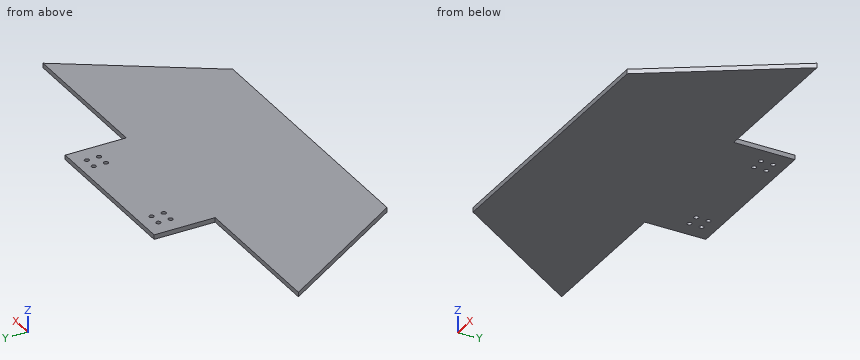
```python
from build123d import *

# Parameters (mm, degrees)
EXTRUDE_1_DEPTH     = 3
CUT_EXTRUDE_1_DEPTH = 10
SKETCH_3_R          = 1.5
CUT_EXTRUDE_2_DEPTH = 10


with BuildPart() as part:
    # 草图1 → 凸台-拉伸1 (new body)
    with BuildSketch(Plane.XY):
        Polygon((100, 0), (250, 0), (250, -30), (330.569672928, -30), (265, -131.238140798), (85, -131.238140798), (19.430327072, -30), (100, -30), align=None)
    extrude(amount=EXTRUDE_1_DEPTH)

    # 草图2 → 切除-拉伸1 (cut)
    with BuildSketch(Plane.XY.offset(3)):
        Polygon((250, -40), (324.092897238, -40), (330.569672928, -30), (250, -30), (250, 0), (226.9, 0), (226.9, -40), align=None)
        Polygon((100, -40), (25.907102762, -40), (19.430327072, -30), (100, -30), (100, 0), (123.1, 0), (123.1, -40), align=None)
    extrude(amount=-CUT_EXTRUDE_1_DEPTH, mode=Mode.SUBTRACT)

    # 草图3 → 切除-拉伸2 (cut)
    with BuildSketch(Plane.XY.offset(3)):
        with Locations((134.1, -9)):
            Circle(SKETCH_3_R)
        with Locations((134.1, -17)):
            Circle(SKETCH_3_R)
        with Locations((142.1, -9)):
            Circle(SKETCH_3_R)
        with Locations((142.1, -17)):
            Circle(SKETCH_3_R)
        with Locations((207.9, -8)):
            Circle(SKETCH_3_R)
        with Locations((215.9, -8)):
            Circle(SKETCH_3_R)
        with Locations((207.9, -16)):
            Circle(SKETCH_3_R)
        with Locations((215.9, -16)):
            Circle(SKETCH_3_R)
    extrude(amount=-CUT_EXTRUDE_2_DEPTH, mode=Mode.SUBTRACT)


solid = part.part
```
Geometry check sheet. Reference: the model listing, model coordinates, mm. Round coordinates to 2 decimals unless told otherwise and drop trailing zeros. Order: outer loops, then holes, each group sorted by start corner. A loop starts at its lowest first (then second) coordinate and runs counter-clockwise, first axis right, second up. Notation, with made-up numbers: (88.5, 33) -> (121.5, 33) arc R19 cw to (121.5, 53) -> close; hole circle Ø7 at (27, 67). An arc over 180 degrees is marked (long way). Return JSON: item names as keys, results as strings. Group by question number.
Q1. Material ranges on probe 1 along Y at (x, z) = (142.1, 2.15); probe 2 along Y at (x, z) = (134.5, 2.7); probe 3 along X at (y, z) = (-31, 0.4), recorded low to high. Write a range as from..to.
Q2. Gauge pin test, flat ends, axial feed: pin 1 (2.5 mm diameter, centred on x = 215.9, y = -16, fed in from -Z); pin 2 (3.5 mm diameter, centred on x = 207.9, y = -8, fed in from -Z); pin 3 (1.5 mm diameter, centred on y = -107.5, z = 1, fed in from +X); pin 4 (1.5 mm diameter, centred on y = -25, z = 2, fed in from +X). Record the tip position at first contact, or that the pin passes through.
Q3. Section check C-C, the plane y = -51. Record the boundary of the cut face in (x, z).
Q4. Section check B-B, the plane y = -27. Record the boundary of the cut face in (x, z), plus the area to 3 significant figures.
Q5. Section check A-A, the plane z = 1.8. Count the separate pieces of the cut face and the enclosed holes in it, plus the area to 3 significant figures.
Numbers:
{
 "1": {"probe 1": "-131.24..-18.5, -15.5..-10.5, -7.5..0", "probe 2": "-131.24..-18.45, -15.55..-10.45, -7.55..0", "probe 3": "123.1..226.9"},
 "2": {"pin 1": "through", "pin 2": "z = 0", "pin 3": "x = 280.86", "pin 4": "x = 226.9"},
 "3": {"outline": "(33.03, 0) -> (316.97, 0) -> (316.97, 3) -> (33.03, 3) -> close"},
 "4": {"outline": "(123.1, 0) -> (226.9, 0) -> (226.9, 3) -> (123.1, 3) -> close", "area": "311 mm^2"},
 "5": {"separate pieces": "1", "enclosed holes": "8", "area": "25,900 mm^2"}
}
